```python
from build123d import *

# Parameters (mm, degrees)
SKIZZE1_R                         = 10
AUFSATZ_LINEAR_AUSTRAGEN1_DEPTH   = 1
SKIZZE2_R                         = 30
AUFSATZ_LINEAR_AUSTRAGEN2_DEPTH   = 2
AUFSATZ_LINEAR_AUSTRAGEN3_DEPTH   = 1
AUFSATZ_LINEAR_AUSTRAGEN3_2_DEPTH = 1
SKIZZE4_R                         = 10
AUFSATZ_LINEAR_AUSTRAGEN4_DEPTH   = 1
AUFSATZ_LINEAR_START              = 3
AUFSATZ_LINEAR_AUSTRAGEN15_DEPTH  = 3


with BuildPart() as part:
    # Skizze1 → Aufsatz-Linear austragen1 (new body)
    with BuildSketch(Plane(origin=(0, 0, 0), x_dir=(1, 0, 0), z_dir=(0, 1, 0))):
        with Locations(Location((0, 0, 0), (0, 0, 270))):
            Circle(SKIZZE1_R)
    extrude(amount=-AUFSATZ_LINEAR_AUSTRAGEN1_DEPTH)

    # Skizze2 → Aufsatz-Linear austragen2 (add)
    with BuildSketch(Plane(origin=(0, 0, 0), x_dir=(1, 0, 0), z_dir=(0, 1, 0))):
        with Locations(Location((0, 0, 0), (0, 0, 270))):
            Circle(SKIZZE2_R)
    extrude(amount=AUFSATZ_LINEAR_AUSTRAGEN2_DEPTH)



with BuildPart() as body_2:
    # Skizze3 → Aufsatz-Linear austragen3 (new body)
    with BuildSketch(Plane.XZ.offset(1)):
        with BuildLine():
            Line((-7.071067812, 7.071067812), (-9.192388155, 9.192388155))
            ThreePointArc((-9.192388155, 9.192388155), (-13, 0), (-9.192388155, -9.192388155))
            Line((-9.192388155, -9.192388155), (-7.071067812, -7.071067812))
            ThreePointArc((-7.071067812, -7.071067812), (-10, 0), (-7.071067812, 7.071067812))
        make_face()
    extrude(amount=AUFSATZ_LINEAR_AUSTRAGEN3_DEPTH)


with BuildPart() as body_3:
    # Skizze3 → Aufsatz-Linear austragen3 2 (new body)
    with BuildSketch(Plane.XZ.offset(1)):
        with BuildLine():
            Line((7.071067812, 7.071067812), (9.192388155, 9.192388155))
            ThreePointArc((9.192388155, 9.192388155), (13, 0), (9.192388155, -9.192388155))
            Line((9.192388155, -9.192388155), (7.071067812, -7.071067812))
            ThreePointArc((7.071067812, -7.071067812), (10, 0), (7.071067812, 7.071067812))
        make_face()
    extrude(amount=AUFSATZ_LINEAR_AUSTRAGEN3_2_DEPTH)


with BuildPart() as part_1:
    add(part.part)

    add(body_2.part)  # Aufsatz-Linear austragen4 merges body 2

    add(body_3.part)  # Aufsatz-Linear austragen4 merges body 3
    # Skizze4 → Aufsatz-Linear austragen4 (add)
    with BuildSketch(Plane.XZ.offset(1)):
        with Locations(Location((0, 0, 0), (0, 0, 90))):
            Circle(SKIZZE4_R)
    extrude(amount=AUFSATZ_LINEAR_AUSTRAGEN4_DEPTH)

    # Skizze8 → Aufsatz-Linear austragen15 (add)
    with BuildSketch(Plane(origin=(0, -1, 0), x_dir=(1, 0, 0), z_dir=(0, 1, 0)).offset(AUFSATZ_LINEAR_START)):
        with BuildLine():
            Line((10.076521944, -8.213629254), (7.737557516, -6.334840462))
            ThreePointArc((7.737557516, -6.334840462), (7.413457608, -6.711232845), (7.071067812, -7.071067812))
            Line((7.071067812, -7.071067812), (9.192388155, -9.192388155))
            ThreePointArc((9.192388155, -9.192388155), (9.646875989, -8.714228804), (10.076521944, -8.213629254))
        make_face()
        with BuildLine():
            Line((-7.071067812, 7.071067812), (-9.192388155, 9.192388155))
            ThreePointArc((-9.192388155, 9.192388155), (-9.636776415, 8.725396284), (-10.057468336, 8.236949111))
            Line((-10.057468336, 8.236949111), (-7.732766819, 6.340687449))
            ThreePointArc((-7.732766819, 6.340687449), (-7.410920578, 6.714034271), (-7.071067812, 7.071067812))
        make_face()
    extrude(amount=-AUFSATZ_LINEAR_AUSTRAGEN15_DEPTH)


solid = part_1.part
```
Can you work these out from the model? Positions are in its coordinate system, mm. A direction names the side the tool comes from. Coordinates: 2 decimals unless noted, no trailing zeros. Loops run counter-clockwise (first coordinate to the right, second up) from the corner with the lowest first, then second, coordinate; pieces in that order, holes last. Notation, with made-up numbers: M 63.25,35.5 L 81.25,35.5 A16 cw 81.25,41.5 Z; hole C 38,80 d6. An arc over 180 degrees is marked long. Put each result on its own line as item: value. Start each with the question number.
(1) Imagine slicing it at C-C on y = 1.1. List the corners of the cut face in (x, z) for me.
(2) Imagine slicing it at D-D on x = 24. List the corners of the cut face in (y, z) for me, and give its area (3 significant figures).
(3) I need wall thicknesses on probe 1 along Y at (x, z) = (4, -10.5); probe 2 along X at (y, z) = (-1.5, -7.5); probe 3 along X at (y, z) = (-0.45, -8). Which ranges of each line are inside material? Lowest first, please.
(4) Will this pin go through, and if not, where does the flat tip stop? pin 1 Ø8 at (x, z) = (-21, -7.5) entering from -Y.
(5) Imagine slicing it at A-A on x = 0. List the corners of the cut face in (y, z) for me, and give its area (3 significant figures).
(6) Which directions (+Z, -Z, +X, -X, +Y, -Y) give clear straight access to the entire face, cutting with the end or side of a thin tool? Please do faces 1 (the face through (-4.071, -0.764, 9.134)), 2 (the face through (-8.1, -1.5, 8.1)), 3 (the face through (1.32, 0.99, -29.97)), 4 (the face through (8.923, -0.493, 7.287)), 5 (the face through (8.1, -1.5, -8.1)).
(7) We'd pull the mould along Z, two halves only. Please class faces 6 (the face through (-8.91, -0.49, -7.3)), 7 (the face through (-8, -1, -8)), 8 (the face through (0, 2, 0)): +Z half, -Z half, draft (parallel to the pull), parting line (faces both ways), or undercut.
(8) Imagine slicing it at B-B on z = 0. List the corners of the cut face in (x, y) for me, and give its area (3 significant figures).
Worked answers:
1. outline: C 0,0 d60
2. outline: M 0,-18 L 2,-18 L 2,18 L 0,18 Z
2. area: 72.0 mm2
3. probe 1: y = 0 to 2
3. probe 2: x = -10.62 to -7.5, -6.61 to 6.61, 7.5 to 10.62
3. probe 3: x = -9.77 to -8, -6 to 6
4. pin 1: stops at y = 0
5. outline: M -2,-10 L 0,-10 L 0,-30 L 2,-30 L 2,30 L 0,30 L 0,10 L -2,10 Z
5. area: 160 mm2
6. face 1: none
6. face 2: +Z, -Y
6. face 3: +Y, -Y
6. face 4: +X
6. face 5: -Z, -Y
7. face 6: undercut
7. face 7: -Z half
7. face 8: draft
8. outline: M -30,0 L -10,0 L -10,-1 L -13,-1 L -13,-2 L 13,-2 L 13,-1 L 10,-1 L 10,0 L 30,0 L 30,2 L -30,2 Z
8. area: 166 mm2
